from build123d import *

# Parameters (mm, degrees)
F0_W     = 30
F0_H     = 6
F1_DEPTH = 3
F2_R     = 2.4
F2_R_2   = 1.25
F3_DEPTH = 2.5
F4_DEPTH = 3.001
F5_R     = 2.99999
F6_SIZE  = 0.4


# Not quite as in the source:
# - a fillet or chamfer is up to 0.001 mm smaller than in the source, because OpenCascade refuses the exact size


with BuildPart() as f1:
    # F0 (on Top) → F1 (new body)
    with BuildSketch(Plane.XY):
        with Locations((15, 0)):
            Rectangle(F0_W, F0_H)
    extrude(amount=F1_DEPTH)

    # F2 (on face) → F3 (cut)
    with BuildSketch(Plane(origin=(0, 0, 0), x_dir=(1, 0, 0), z_dir=(0, 0, -1))):
        with Locations((3.4, 0)):
            Circle(F2_R)
        with Locations((3.4, 0)):
            Circle(F2_R_2, mode=Mode.SUBTRACT)
        with Locations((3.4, 0)):
            Circle(F2_R_2)
    extrude(amount=-F3_DEPTH, mode=Mode.SUBTRACT)

    # F2 (on face) → F4 (cut, through all)
    with BuildSketch(Plane(origin=(0, 0, 0), x_dir=(1, 0, 0), z_dir=(0, 0, -1))):
        with Locations((3.4, 0)):
            Circle(F2_R_2)
    extrude(amount=-F4_DEPTH, mode=Mode.SUBTRACT)

    # F5 (radius 3 in the source; OpenCascade refuses exactly that, so slightly less here)
    f5_edges = [f1.edges().sort_by_distance(p)[0] for p in [
        (0, -3, 1.5),
        (0, 3, 1.5),
        (30, -3, 1.5),
        (30, 3, 1.5),
    ]]
    fillet(f5_edges, radius=F5_R)

    # F6
    f6_edges = [f1.edges().sort_by_distance(p)[0] for p in [
        (15, 3, 3),
    ]]
    chamfer(f6_edges, length=F6_SIZE)


solid = f1.part
Read the model definition and answer for the solid it produces. Units are mm, in the model's axes. A direction names the side the tool comes from. Round coordinates to 2 decimals unless told otherwise and drop trailing zeros. Order: outer loops, then holes, each group sorted by start corner. A loop starts at its lowest first (then second) coordinate and runs counter-clockwise, first axis right, second up. Notation, with made-up numbers: (75, -8.5) - (80, -8.5) arc R29 cw to (80, 18.5) - close; hole circle Ø8 at (-26, 82). An arc over 180 degrees is marked (long way). Use one line per item in the form item = value. Start each with the question number.
(1) The part is cut by section A-A (x = 3.4). Give the vertices of the cut face in (y, z).
(2) For faces 1 (the face through (4.555, 0.479, 2.746)), 2 (the face through (4.69, -2.024, 1.232)), determine the directions among +Z, -Z, +X, -X, +Y, -Y from which every point of the face is accessible in a straight line to the end or side of a thin tool.
(3) Flat-ended cylindrical pins translate along their axes: pin 1 Ø1.5 at (y, z) = (-2, 2.5) entering from +X; pin 2 Ø2 at (x, y) = (3.4, 0) entering from -Z; pin 3 Ø1 at (y, z) = (-1, 1) entering from +X. Find the tip coordinate at first contact, or state that the pin passes through.
(4) Determine the mould class of faces 3 (the face through (28.94, -1.898, 2.886)), 4 (the face through (1.06, 1.898, 2.886)), 5 (the face through (4.4, 1, 2.5)) for opening direction Y: +Y half, -Y half, draft (parallel to the pull), parting line (faces both ways), or undercut.
(5) Find the intervals of material crossed by line 1 along X through (y, z) = (0, 1.75); line 2 along Y through (x, z) = (3.4, 1.85); line 3 along Y through (x, z) = (4.25, 1.2), in increasing order. Write a range as from..to.
Checked values:
q1.outline = (-3, 0) - (-2.4, 0) - (-2.4, 2.5) - (-1.25, 2.5) - (-1.25, 3) - (-2.6, 3) - (-3, 2.6) - close; (1.25, 2.5) - (2.4, 2.5) - (2.4, 0) - (3, 0) - (3, 2.6) - (2.6, 3) - (1.25, 3) - close
q2.face_1 = +Z, -Z
q2.face_2 = -Z
q3.pin_1 = 29.73
q3.pin_2 = through
q3.pin_3 = 29.96
q4.face_3 = -Y half
q4.face_4 = +Y half
q4.face_5 = undercut
q5.line_1 = 0..1, 5.8..30
q5.line_2 = -3..-2.4, 2.4..3
q5.line_3 = -3..-2.24, 2.24..3
